Read the model definition and answer for the solid it produces. Units are mm, in the model's axes. A direction names the side the tool comes from. Coordinates: 2 decimals unless noted, no trailing zeros. Write each loop counter-clockwise with the first axis right and the second up, starting at its lowest first coordinate (ties: lowest second). Pieces come first, ordered by that corner, then holes. Notation, with made-up numbers: M 62.5,-31 L 92.5,-31 A24 ccw 92.5,-16 Z; hole C -8,59.5 d4. An arc over 180 degrees is marked long. Write item = value, one per line.
from build123d import *

# Parameters (mm, degrees)
F0_R     = 30
F1_DEPTH = 4
F2_R     = 28.075
F3_DEPTH = 14.4
F4_R     = 23.5
F5_DEPTH = 14
F6_R     = 15
F7_DEPTH = 18.401


with BuildPart() as f1:
    # F0 (on Top) → F1 (new body)
    with BuildSketch(Plane.XY):
        Circle(F0_R)
    extrude(amount=F1_DEPTH)

    # F2 (on face) → F3 (join)
    with BuildSketch(Plane.XY.offset(4)):
        Circle(F2_R)
    extrude(amount=F3_DEPTH)

    # F4 (on face) → F5 (cut)
    with BuildSketch(Plane(origin=(0, 0, 0), x_dir=(1, 0, 0), z_dir=(0, 0, -1))):
        Circle(F4_R)
    extrude(amount=-F5_DEPTH, mode=Mode.SUBTRACT)

    # F6 (on face) → F7 (cut, through all)
    with BuildSketch(Plane.XY.offset(18.4)):
        Circle(F6_R)
    extrude(amount=-F7_DEPTH, mode=Mode.SUBTRACT)


solid = f1.part
Item 1: For a pull along Y with two mould halves and no side action, classify faces 3 (the face through (20, -20, 4)), 4 (the face through (-0.3, 15.3, 14)), 5 (the face through (26.78, 8.43, 11.1)) as released by +Y, released by -Y, zero draft, split by the parting line, or undercut.
Worked answers:
face_3 = zero draft
face_4 = undercut
face_5 = split by the parting line
Item 2: Find section D-D (y = -20). Determine the outline of the cut face in (x, z), and give its area (3 significant figures).
Worked answers:
outline = M -22.36,0 L -12.34,0 L -12.34,14 L 12.34,14 L 12.34,0 L 22.36,0 L 22.36,4 L 19.7,4 L 19.7,18.4 L -19.7,18.4 L -19.7,4 L -22.36,4 Z
area = 401 mm²
Item 3: Flat-ended cylindrical pins translate along their axes: pin 1 (1 mm diameter, centred on x = -18.5, z = 14.5, fed in from -Y); pin 2 (1 mm diameter, centred on x = -8, z = 13.5, fed in from -Y). Find the tip coordinate at first contact, or state that the pin passes through.
Worked answers:
pin_1 = -21.55
pin_2 = -27.05
Item 4: Which of the six approach directions +Z, -Z, +X, -X, +Y, -Y give full straight-line access (tool end or side, diameter ignored) to faces 1 (the face through (12, -12, 18.4)), 2 (the face through (22.4, -7.1, 6.9))?
Worked answers:
face_1 = +Z, +X, -X, +Y, -Y
face_2 = -Z
Item 5: Consider line 1 along Y through (x, z) = (0, 16.95) (3 decimals); line 2 along X through (y, z) = (-0.5, 3); line 3 along Y through (x, z) = (0, 3.5). Determine where each line is inside the solid, lowest interval first. Write a range as from..to.
Worked answers:
line_1 = -28.075..-15, 15..28.075
line_2 = -30..-23.49, 23.49..30
line_3 = -30..-23.5, 23.5..30
Item 6: Find section C-C (z = 7.5). Determine the outline of the cut face in (x, y) (3 decimals), and give its area (3 significant figures).
Worked answers:
outline = C 0,0 d56.15; hole C 0,0 d47
area = 741 mm²
Item 7: Find section A-A (y = 0). Determine the outline of the cut face in (x, z) (3 decimals), and give its area (3 significant figures).
Worked answers:
outline = M -30,0 L -23.5,0 L -23.5,14 L -15,14 L -15,18.4 L -28.075,18.4 L -28.075,4 L -30,4 Z; M 15,14 L 23.5,14 L 23.5,0 L 30,0 L 30,4 L 28.075,4 L 28.075,18.4 L 15,18.4 Z
area = 259 mm²
